Here's how the part is built. I have some questions about the finished solid (model axes, mm). Coordinates: 2 decimals unless noted, no trailing zeros. Order: outer loops, then holes, each group sorted by start corner. A loop starts at its lowest first (then second) coordinate and runs counter-clockwise, first axis right, second up. Notation, with made-up numbers: (7.5, 11) - (48.5, 11) arc R24 ccw to (48.5, 21) - close; hole circle Ø7 at (-30.5, 77). An arc over 180 degrees is marked (long way). Answer in a Markdown table with one row per item. Add a question column.
Item 1: I want a section at C-C (x = 1.5). Please give me the cut outline in (y, z), plus the area to 3 significant figures.
Item 2: I want a section at B-B (x = -4). Please give me the cut outline in (y, z).
Item 3: I want a section at A-A (y = -0.25). Please give me the cut outline in (x, z).
Item 4: If I drill on line 1 along Y through (x, z) = (3.25, -2.4); line 2 along X through (y, z) = (0.75, -0.9); line 3 along Y through (x, z) = (-4, -0.2), over which ranges is the centre line in solid material (lowest first)? Write a range as from..to.
Item 5: Thinking about a two-plate mould opening in Y: for faces 1 (the cylindrical face through (2.276, -3.284, 0.042)), 2 (the cylindrical face through (-3.21, -2.34, 0.04)), 3 (the flat face through (-1.1, 0.1, -3)), which applies, +Y half, -Y half, draft (parallel to the pull), parting line (faces both ways), or undercut?
Item 6: Will these pins go through, and if not, where does the flat tip stop? pin 1 Ø3 at (y, z) = (-3, -1) entering from +X; pin 2 Ø3 at (x, z) = (0, -1) entering from -Y; pin 3 Ø1 at (x, z) = (3.5, 0.5) entering from +Y.
```python
from build123d import *

# Parameters (mm, degrees)
SKETCH1_R           = 6
SKETCH1_R_2         = 0.9
BOSS_EXTRUDE1_DEPTH = 3
SKETCH2_R           = 6
CUT_EXTRUDE1_DEPTH  = 11.392304845


with BuildPart() as part:
    # Sketch1 → Boss-Extrude1 (new, symmetric)
    with BuildSketch(Plane.XY):
        Circle(SKETCH1_R)
        Circle(SKETCH1_R_2, mode=Mode.SUBTRACT)
    extrude(amount=BOSS_EXTRUDE1_DEPTH, both=True)

    # Sketch2 → Cut-Extrude1 (cut, through all)
    with BuildSketch(Plane.XY.offset(3)):
        Circle(SKETCH2_R)
        with BuildLine():
            ThreePointArc((-0.904303163, 2.859411966), (-1.23929318, 3.784776039), (-2.052505646, 4.339034521))
            ThreePointArc((-2.052505646, 4.339034521), (-2.138842368, 4.297133152), (-2.224324134, 4.253514094))
            ThreePointArc((-2.224324134, 4.253514094), (-2.272407373, 3.270556831), (-1.736096974, 2.44539737))
            ThreePointArc((-1.736096974, 2.44539737), (-2.100579038, 2.140459929), (-2.412316811, 1.781776811))
            ThreePointArc((-2.412316811, 1.781776811), (-3.227244783, 2.333509881), (-4.210932449, 2.303920118))
            ThreePointArc((-4.210932449, 2.303920118), (-4.256151318, 2.219273746), (-4.29966888, 2.133740266))
            ThreePointArc((-4.29966888, 2.133740266), (-3.760801254, 1.310248516), (-2.841900466, 0.957915832))
            ThreePointArc((-2.841900466, 0.957915832), (-2.957534919, 0.496979078), (-2.998907428, 0.023563475))
            ThreePointArc((-2.998907428, 0.023563475), (-3.982498568, -0.009077739), (-4.760926181, -0.611213463))
            ThreePointArc((-4.760926181, -0.611213463), (-4.747755125, -0.706272801), (-4.732686255, -0.801049821))
            ThreePointArc((-4.732686255, -0.801049821), (-3.812696882, -1.150530198), (-2.862194572, -0.895456995))
            ThreePointArc((-2.862194572, -0.895456995), (-2.684812984, -1.336330888), (-2.440017337, -1.743650307))
            ThreePointArc((-2.440017337, -1.743650307), (-3.216573261, -2.348197971), (-3.49240793, -3.292884275))
            ThreePointArc((-3.49240793, -3.292884275), (-3.425877845, -3.362047143), (-3.357978338, -3.429866103))
            ThreePointArc((-3.357978338, -3.429866103), (-2.408271889, -3.171845481), (-1.789227635, -2.406795685))
            ThreePointArc((-1.789227635, -2.406795685), (-1.386583742, -2.659207876), (-0.949123556, -2.844848937))
            ThreePointArc((-0.949123556, -2.844848937), (-1.222026295, -3.79038639), (-0.889908552, -4.716785215))
            ThreePointArc((-0.889908552, -4.716785215), (-0.795431669, -4.733633748), (-0.700636829, -4.74859011))
            ThreePointArc((-0.700636829, -4.74859011), (-0.083968889, -3.981623598), (-0.032836554, -2.998820228))
            ThreePointArc((-0.032836554, -2.998820228), (0.44127336, -2.966357838), (0.904303163, -2.859411966))
            ThreePointArc((0.904303163, -2.859411966), (1.23929318, -3.784776039), (2.052505646, -4.339034521))
            ThreePointArc((2.052505646, -4.339034521), (2.138842368, -4.297133152), (2.224324134, -4.253514094))
            ThreePointArc((2.224324134, -4.253514094), (2.272407373, -3.270556831), (1.736096974, -2.44539737))
            ThreePointArc((1.736096974, -2.44539737), (2.100579038, -2.140459929), (2.412316811, -1.781776811))
            ThreePointArc((2.412316811, -1.781776811), (3.227244783, -2.333509881), (4.210932449, -2.303920118))
            ThreePointArc((4.210932449, -2.303920118), (4.256151318, -2.219273746), (4.29966888, -2.133740266))
            ThreePointArc((4.29966888, -2.133740266), (3.760801254, -1.310248516), (2.841900466, -0.957915832))
            ThreePointArc((2.841900466, -0.957915832), (2.957534919, -0.496979078), (2.998907428, -0.023563475))
            ThreePointArc((2.998907428, -0.023563475), (3.982498568, 0.009077739), (4.760926181, 0.611213463))
            ThreePointArc((4.760926181, 0.611213463), (4.747755125, 0.706272801), (4.732686255, 0.801049821))
            ThreePointArc((4.732686255, 0.801049821), (3.812696882, 1.150530198), (2.862194572, 0.895456995))
            ThreePointArc((2.862194572, 0.895456995), (2.684812984, 1.336330888), (2.440017337, 1.743650307))
            ThreePointArc((2.440017337, 1.743650307), (3.216573261, 2.348197971), (3.49240793, 3.292884275))
            ThreePointArc((3.49240793, 3.292884275), (3.425877845, 3.362047143), (3.357978338, 3.429866103))
            ThreePointArc((3.357978338, 3.429866103), (2.408271889, 3.171845481), (1.789227635, 2.406795685))
            ThreePointArc((1.789227635, 2.406795685), (1.386583742, 2.659207876), (0.949123556, 2.844848937))
            ThreePointArc((0.949123556, 2.844848937), (1.222026295, 3.79038639), (0.889908552, 4.716785215))
            ThreePointArc((0.889908552, 4.716785215), (0.795431669, 4.733633748), (0.700636829, 4.74859011))
            ThreePointArc((0.700636829, 4.74859011), (0.083968889, 3.981623598), (0.032836554, 2.998820228))
            ThreePointArc((0.032836554, 2.998820228), (-0.44127336, 2.966357838), (-0.904303163, 2.859411966))
        make_face(mode=Mode.SUBTRACT)
    extrude(amount=-CUT_EXTRUDE1_DEPTH, mode=Mode.SUBTRACT)


solid = part.part
```
Values follow:
| question | item | result |
|---|---|---|
| 1 | outline | (-4.05, -3) - (2.6, -3) - (2.6, 3) - (-4.05, 3) - close |
| 1 | area | 39.9 mm^2 |
| 2 | outline | (-1.13, -3) - (-0.02, -3) - (-0.02, 3) - (-1.13, 3) - close; (1.55, -3) - (2.36, -3) - (2.36, 3) - (1.55, 3) - close |
| 3 | outline | (-4.42, -3) - (-0.86, -3) - (-0.86, 3) - (-4.42, 3) - close; (0.86, -3) - (2.99, -3) - (2.99, 3) - (0.86, 3) - close |
| 4 | line 1 | y = -2.34..-1.03, -0.07..1.08, 2.4..3.43 |
| 4 | line 2 | x = -2.9..-0.5, 0.5..4.74 |
| 4 | line 3 | y = -1.13..-0.02, 1.55..2.36 |
| 5 | face 1 | undercut |
| 5 | face 2 | undercut |
| 5 | face 3 | draft |
| 6 | pin 1 | stops at x = 4.3 |
| 6 | pin 2 | stops at y = -4.75 |
| 6 | pin 3 | stops at y = 3.43 |
